Check sheet for the modelled part. Datum: model origin and axes. Units: mm. A direction names the side the tool comes from. Coordinates: 2 decimals unless noted, no trailing zeros. Write each loop counter-clockwise with the first axis right and the second up, starting at its lowest first coordinate (ties: lowest second). Pieces come first, ordered by that corner, then holes. Notation, with made-up numbers: (-21, 4) -> (16, 4) arc R23 cw to (16, 17) -> close; hole circle Ø7 at (62, 52). An arc over 180 degrees is marked (long way). Put each result on its own line as item: value.
```python
from build123d import *

# Parameters (mm, degrees)
BOSS_EXTRUDE1_DEPTH = 2.5
SKETCH2_R           = 1.1
SKETCH2_R_2         = 1.25
CUT_EXTRUDE1_DEPTH  = 21.81201576
FILLET3_RADIUS      = 2.5
FILLET3_LENGTH      = 2.8
FILLET4_RADIUS      = 2.5
FILLET4_LENGTH      = 2.8
FILLET5_RADIUS      = 2.5
FILLET5_LENGTH      = 4
FILLET6_R           = 2
FILLET7_R           = 2
FILLET8_R           = 1


with BuildPart() as part:
    # Sketch1 → Boss-Extrude1 (new, symmetric)
    with BuildSketch(Plane(origin=(0, 0, 0), x_dir=(1, 0, 0), z_dir=(0, 1, 0))):
        Polygon((11.5, 2), (-11.5, 2), (-11.5, 4.6), (-18.5, 4.6), (-18.5, 1.8), (-13.5, 1.8), (-13.5, -1.8), (-18.5, -1.8), (-18.5, -4.6), (-11.5, -4.6), (-11.5, -2), (11.5, -2), align=None)
    extrude(amount=BOSS_EXTRUDE1_DEPTH, both=True)

    # Sketch2 → Cut-Extrude1 (cut, through all)
    with BuildSketch(Plane.XY.offset(4.6)):
        with Locations((-16, 0)):
            Circle(SKETCH2_R)
        with Locations((9, 0)):
            Circle(SKETCH2_R_2)
    extrude(amount=-CUT_EXTRUDE1_DEPTH, mode=Mode.SUBTRACT)

    # Fillet3: full round fillet: the end face becomes a half cylinder, R = half its width
    fillet3_face = Plane((-18.5, 0, -3.2), x_dir=(0, 0, 1), z_dir=(-1, 0, 0))  # on the end face: x along it, z out of the body
    fillet3_slab = fillet3_face.offset(-FILLET3_RADIUS / 2) * Box(FILLET3_LENGTH, 2 * FILLET3_RADIUS, FILLET3_RADIUS, mode=Mode.PRIVATE)  # the body's end, R deep
    fillet3_round = Plane((-16, 0, -3.2), x_dir=(-1, 0, 0), z_dir=(0, 0, 1)) * Cylinder(FILLET3_RADIUS, FILLET3_LENGTH, mode=Mode.PRIVATE)  # its axis R under the face
    add(fillet3_slab - fillet3_round, mode=Mode.SUBTRACT)

    # Fillet4: full round fillet: the end face becomes a half cylinder, R = half its width
    fillet4_face = Plane((-18.5, 0, 3.2), x_dir=(0, 0, 1), z_dir=(-1, 0, 0))  # on the end face: x along it, z out of the body
    fillet4_slab = fillet4_face.offset(-FILLET4_RADIUS / 2) * Box(FILLET4_LENGTH, 2 * FILLET4_RADIUS, FILLET4_RADIUS, mode=Mode.PRIVATE)  # the body's end, R deep
    fillet4_round = Plane((-16, 0, 3.2), x_dir=(-1, 0, 0), z_dir=(0, 0, 1)) * Cylinder(FILLET4_RADIUS, FILLET4_LENGTH, mode=Mode.PRIVATE)  # its axis R under the face
    add(fillet4_slab - fillet4_round, mode=Mode.SUBTRACT)

    # Fillet5: full round fillet: the end face becomes a half cylinder, R = half its width
    fillet5_face = Plane((11.5, 0, 0), x_dir=(0, 0, 1), z_dir=(1, 0, 0))  # on the end face: x along it, z out of the body
    fillet5_slab = fillet5_face.offset(-FILLET5_RADIUS / 2) * Box(FILLET5_LENGTH, 2 * FILLET5_RADIUS, FILLET5_RADIUS, mode=Mode.PRIVATE)  # the body's end, R deep
    fillet5_round = Plane((9, 0, 0), x_dir=(1, 0, 0), z_dir=(0, 0, 1)) * Cylinder(FILLET5_RADIUS, FILLET5_LENGTH, mode=Mode.PRIVATE)  # its axis R under the face
    add(fillet5_slab - fillet5_round, mode=Mode.SUBTRACT)

    # Fillet6
    fillet6_edges = [part.edges().sort_by_distance(p)[0] for p in [
        (-11.5, 0, 4.6),
    ]]
    fillet(fillet6_edges, radius=FILLET6_R)

    # Fillet7
    fillet7_edges = [part.edges().sort_by_distance(p)[0] for p in [
        (-11.5, 0, -4.6),
    ]]
    fillet(fillet7_edges, radius=FILLET7_R)

    # Fillet8
    fillet8_edges = [part.edges().sort_by_distance(p)[0] for p in [
        (-13.5, -2.5, 0),
        (-13.5, 2.5, 0),
    ]]
    fillet(fillet8_edges, radius=FILLET8_R)


solid = part.part
```
Q1. Material ranges on line 1 along Z through (x, y) = (-15.75, -1.45); line 2 along Y through (x, z) = (-16, 3.7); line 3 along Z through (x, y) = (1.25, 0.85), recorded low to high.
Recorded:
line 1: z = -4.6 to -1.8, 1.8 to 4.6
line 2: y = -2.5 to -1.1, 1.1 to 2.5
line 3: z = -2 to 2
Q2. Cross-section at D-D (x = -10.75). Record the cut outline in (y, z).
Recorded:
outline: (-2.5, -2) -> (2.5, -2) -> (2.5, 2) -> (-2.5, 2) -> close
Q3. Cross-section at C-C (z = 4.25). Record the cut outline in (x, y), plus the area to 3 significant figures.
Recorded:
outline: (-16, -2.5) -> (-12.37, -2.5) -> (-12.37, 2.5) -> (-16, 2.5) arc R2.5 ccw to start; hole circle Ø2.2 at (-16, 0)
area: 24.2 mm2
Q4. Mould release check, pull along Z, two halves, no side actions. Record for faces 5 (the flat face through (-15, 1, -1.8)), 6 (the cylindrical face through (-17.1, 0, -3.2)), 7 (the flat face through (-15, -1, -4.6)), 8 (the cylindrical face through (-13.215, 2.199, 0.025)): released by +Z, released by -Z, zero draft, split by the parting line, or undercut.
Recorded:
face 5: undercut
face 6: zero draft
face 7: released by -Z
face 8: undercut
Q5. Cross-section at A-A (y = 0). Record the cut outline in (x, z), plus the area to 3 significant figures.
Recorded:
outline: (-18.5, -4.6) -> (-17.1, -4.6) -> (-17.1, -1.8) -> (-18.5, -1.8) -> close; (-18.5, 1.8) -> (-17.1, 1.8) -> (-17.1, 4.6) -> (-18.5, 4.6) -> close; (-14.9, -4.6) -> (-13.5, -4.6) arc R2 ccw to (-11.5, -2.6) -> (-11.5, -2) -> (7.75, -2) -> (7.75, 2) -> (-11.5, 2) -> (-11.5, 2.6) arc R2 ccw to (-13.5, 4.6) -> (-14.9, 4.6) -> (-14.9, 1.8) -> (-13.5, 1.8) -> (-13.5, -1.8) -> (-14.9, -1.8) -> close; (10.25, -2) -> (11.5, -2) -> (11.5, 2) -> (10.25, 2) -> close
area: 114 mm2
Q6. Depth check by flat-ended pin: P1, Ø2, axis at x = -16, y = 0, coming from the -Z side; P2, Ø1.5, axis at y = 0.5, z = 0.5, coming from the -X side; P3, Ø1.5, axis at x = 2, y = 1, coming from the -Z side. Enter the tip coordinate at first touch or a pass-through.
Recorded:
P1: passes through
P2: stops at x = -13.5
P3: stops at z = -2
Q7. Cross-section at B-B (x = 9.5). Record the cut outline in (y, z).
Recorded:
outline: (-2.45, -2) -> (-1.15, -2) -> (-1.15, 2) -> (-2.45, 2) -> close; (1.15, -2) -> (2.45, -2) -> (2.45, 2) -> (1.15, 2) -> close
Q8. Tool access check on faces 1 (the flat face through (0, 0, 2)), 2 (the flat face through (-13.5, 0, 0)), 3 (the flat face through (0, 0, -2)), 4 (the cylindrical face through (-13.199, -2.215, 0.025)). Record the directions out of +Z, -Z, +X, -X, +Y, -Y that give a thin tool (end or side, any length) a straight path to the whole face; none if there is none.
Recorded:
face 1: +Z, +X, +Y, -Y
face 2: -X, +Y, -Y
face 3: -Z, +X, +Y, -Y
face 4: -X, -Y
